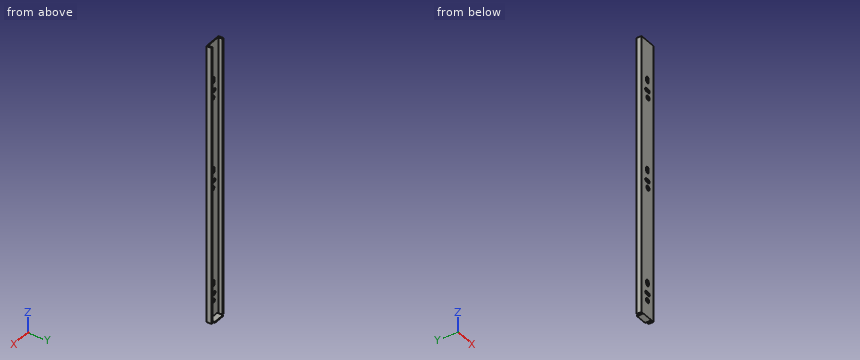
Autodesk Inventor part; units mm, degrees
ref_plane "YZ Plane" through (0, 0, 0) normal (1, 0, 0) x (0, 1, 0)
ref_plane "XZ Plane" through (0, 0, 0) normal (0, 1, 0) x (-1, 0, 0)
ref_plane "XY Plane" through (0, 0, 0) normal (0, 0, 1) x (1, 0, 0)
sketch "Эскиз1" plane through (0, 0, 0) normal (0, 0, 1) x (1, 0, 0)
  line L0 (0, 0) -> (24, 0)
  line L1 (24, 0) -> (24, 7)
  line L2 (24, 7) -> (0, 7)
  line L3 (0, 7) -> (0, 0)
  line L4 (0, 1) -> (24, 1)
  line L5 (2, 7) -> (2, 0)
  line L6 (22, 7) -> (22, 0)
  point P0 (0, 3.5)
  point P1 (12, 0)
  point P2 (2, 1)
  point P3 (22, 1)
  dimension "d0" = 24
  dimension "d1" = 7
  dimension "d2" = 2
  dimension "d3" = 2
  dimension "d4" = 1
extrude "Выдавливание1" add sketch "Эскиз1" along normal blind 390 contours L3 L4 L5 L0 | L5 L4 L6 L0 | L3 L2 L5 L4 | L6 L4 L1 L0 | L6 L2 L1 L4
sketch "Эскиз3" plane through (0, 0, 0) normal (0, -1, 0) x (1, 0, 0)
  line L0 (12.0032, 0) -> (12, 390)
  line L1 (22, 390) -> (2, 390)
  circle A0 centre (12.003, 23) radius 3.25
  line L2 (0, 0) -> (24, 0)
  line L3 (7.5, 33) -> (16.5, 33) construction
  line L4 (24, 0) -> (24, 390)
  line L5 (10, 30.5) -> (14, 30.5)
  line L6 (14, 35.5) -> (10, 35.5)
  arc A1 (10, 35.5) -> (10, 30.5) centre (10, 33) ccw
  arc A2 (14, 30.5) -> (14, 35.5) centre (14, 33) ccw
  line L7 (12.0029, 43.5) -> (12.0028, 52.5) construction
  line L8 (14.5028, 46) -> (14.5028, 50)
  line L9 (9.5028, 50) -> (9.5028, 46)
  arc A3 (9.5028, 46) -> (14.5028, 46) centre (12.0028, 46) ccw
  arc A4 (14.5028, 50) -> (9.5028, 50) centre (12.0028, 50) ccw
  circle A5 centre (12.9217, 182.4968) radius 3.25
  line L10 (7.4336, 192.5395) -> (16.4317, 192.3559) construction
  line L11 (9.8821, 189.989) -> (13.8813, 189.9074)
  line L12 (13.9833, 194.9064) -> (9.9841, 194.988)
  arc A6 (9.9841, 194.988) -> (9.8821, 189.989) centre (9.9331, 192.4885) ccw
  arc A7 (13.8813, 189.9074) -> (13.9833, 194.9064) centre (13.9323, 192.4069) ccw
  line L13 (11.9196, 202.9469) -> (11.9271, 211.9469) construction
  line L14 (14.4217, 205.4448) -> (14.425, 209.4448)
  line L15 (9.425, 209.449) -> (9.4217, 205.449)
  arc A8 (9.4217, 205.449) -> (14.4217, 205.4448) centre (11.9217, 205.4469) ccw
  arc A9 (14.425, 209.4448) -> (9.425, 209.449) centre (11.925, 209.4469) ccw
  line L16 (11.9646, 330.3923) -> (11.9626, 339.3923) construction
  line L17 (14.464, 332.8928) -> (14.4632, 336.8928)
  arc A10 (14.4632, 336.8928) -> (9.4632, 336.8918) centre (11.9632, 336.8923) ccw
  arc A11 (9.464, 332.8918) -> (14.464, 332.8928) centre (11.964, 332.8923) ccw
  line L18 (7.4209, 320.0033) -> (16.4182, 319.7828) construction
  arc A12 (9.9814, 322.4413) -> (9.8589, 317.4428) centre (9.9201, 319.9421) ccw
  circle A13 centre (12.9562, 309.9469) radius 3.25
  line L19 (9.4632, 336.8918) -> (9.464, 332.8918)
  line L20 (13.9802, 322.3433) -> (9.9814, 322.4413)
  arc A14 (13.8577, 317.3448) -> (13.9802, 322.3433) centre (13.9189, 319.844) ccw
  line L21 (9.8589, 317.4428) -> (13.8577, 317.3448)
  point P0 (12, 33)
  point P1 (12.0028, 48)
  point P2 (12, 35.5)
  point P3 (11.9327, 192.4477)
  point P4 (11.9233, 207.4469)
  point P5 (11.9837, 194.9472)
  point P6 (12.0028, 52.5)
  point P7 (11.9636, 334.8923)
  point P8 (11.9646, 330.3923)
  point P9 (11.9195, 319.8931)
  point P10 (11.9808, 322.3923)
  point P11 (11.9271, 211.9469)
  dimension "d7" = 6.5
  dimension "d8" = 23
  dimension "d9" = 9
  dimension "d10" = 5
  dimension "d11" = 10
  dimension "d12" = 9
  dimension "d13" = 5
  dimension "d14" = 8
  dimension "d15" = 6.5
  dimension "d16" = 9
  dimension "d17" = 5
  dimension "d18" = 10
  dimension "d19" = 9
  dimension "d20" = 5
  dimension "d21" = 8
  dimension "d22" = 130
  dimension "d23" = 6.5
  dimension "d24" = 9
  dimension "d25" = 5
  dimension "d26" = 10
  dimension "d27" = 9
  dimension "d28" = 5
  dimension "d29" = 8
  dimension "d30" = 98
extrude "Выдавливание2" cut sketch "Эскиз3" against normal blind 10
sketch "Эскиз4" plane through (0, 0, 0) normal (0, 0, -1) x (-1, 0, 0)
  line L0 (-2, 7) -> (0, 7)
  line L1 (-2, 1) -> (-2, 7)
  line L2 (-22, 1) -> (-2, 1)
  line L3 (-22, 7) -> (-22, 1)
  line L4 (-24, 7) -> (-22, 7)
  line L5 (-24, 0) -> (-24, 7)
  line L6 (0, 0) -> (-24, 0)
  line L7 (0, 7) -> (0, 0)
  line L8 (-12, 9) -> (-20, 9)
  line L9 (-20, 9) -> (-20, 0)
  line L10 (-12, 9) -> (-4, 9)
  line L11 (-4, 9) -> (-4, 0)
  point P0 (-20, 1)
  point P1 (-4, 1)
extrude "Выдавливание3" add sketch "Эскиз4" against normal blind 1.5 contours L2 L9 L8 L10 L11
properties part number "3 часть направляшки"
Verification items for the finished model (mm, model axes). Round coordinates to 2 decimals unless told otherwise and drop trailing zeros. Write each loop counter-clockwise with the first axis right and the second up, starting at its lowest first coordinate (ties: lowest second). Pieces come first, ordered by that corner, then holes. Notation, with made-up numbers: (86, -17) - (141, -17) arc R27 cw to (141, 3) - close; hole circle Ø4 at (23.5, 86). An arc over 180 degrees is marked (long way). Answer as a JSON object with one key per item and string values. Group by question number.
Q1. Thickness scan on line 1 (X direction, y = 6.5, z = 62); line 2 (X direction, y = 0.7, z = 23); line 3 (Y direction, x = 11, z = 105). Record the ranges inside material, lowest first.
Q2. Section check C-C, the plane z = 100.5. Enter the section's corners in (x, y).
Q3. Go/stop test with flat-tipped pins: pin 1 Ø2.5 at (x, y) = (11, 4) entering from +Z; pin 2 Ø10 at (x, z) = (11.5, 292) entering from +Y; pin 3 Ø1.6 at (x, z) = (1, 259.5) entering from +Y. Record where each tip stops, or that it passes through.
Q4. Section check A-A, the plane y = 4. Enter the section's corners in (x, z).
Q5. Section check B-B, the plane z = 23. Enter the section's corners in (x, y), plus the area to 3 significant figures.
Found:
{
 "1": {"line 1": "x = 0 to 2, 22 to 24", "line 2": "x = 0 to 8.75, 15.25 to 24", "line 3": "y = 0 to 1"},
 "2": {"outline": "(0, 0) - (24, 0) - (24, 7) - (22, 7) - (22, 1) - (2, 1) - (2, 7) - (0, 7) - close"},
 "3": {"pin 1": "stops at z = 1.5", "pin 2": "stops at y = 1", "pin 3": "stops at y = 7"},
 "4": {"outline": "(0, 0) - (2, 0) - (2, 390) - (0, 390) - close; (4, 0) - (20, 0) - (20, 1.5) - (4, 1.5) - close; (22, 0) - (24, 0) - (24, 390) - (22, 390) - close"},
 "5": {"outline": "(0, 0) - (8.75, 0) - (8.75, 1) - (2, 1) - (2, 7) - (0, 7) - close; (15.25, 0) - (24, 0) - (24, 7) - (22, 7) - (22, 1) - (15.25, 1) - close", "area": "41.5 mm^2"}
}
